Autodesk Inventor part; units mm, degrees
ref_plane "YZ Plane" through (0, 0, 0) normal (1, 0, 0) x (0, 1, 0)
ref_plane "XZ Plane" through (0, 0, 0) normal (0, 1, 0) x (-1, 0, 0)
ref_plane "XY Plane" through (0, 0, 0) normal (0, 0, 1) x (1, 0, 0)
sketch "Sketch1" plane through (0, 0, 0) normal (0, 0, 1) x (1, 0, 0)
  line L0 (10, -20) -> (-10, -20)
  line L1 (-10, -20) -> (-10, 20)
  line L2 (-10, 20) -> (10, 20)
  line L3 (10, 20) -> (10, -20)
  line L4 (10, -20) -> (-10, 20) construction
  line L5 (-10, -20) -> (10, 20) construction
  line L6 (0, -10) -> (0, 10) construction
  circle A0 centre (0, 10) radius 2.65
  circle A1 centre (0, -10) radius 2.65
  point P0 (0, 0)
  dimension "d0" = 40
  dimension "d1" = 20
  dimension "d2" = 20
  dimension "d3" = 5.3
extrude "Extrusion1" add sketch "Sketch1" along normal blind 3
ref_plane "Work Plane2" through (0, 0, -24) normal (0, 0, -1) x (-1, 0, 0)
sketch "Sketch2" plane through (0, 0, -24) normal (0, 0, -1) x (-1, 0, 0)
  circle A0 centre (18.05, -6.8) radius 1.65
  line L0 (18.05, -25.9) -> (18.05, -6.8) construction
  line L1 (4.6, -29) -> (20.7, -29)
  line L2 (4.6, 11.5) -> (4.6, -29)
  line L3 (20.7, 11.5) -> (4.6, 11.5)
  line L4 (20.7, -29) -> (20.7, 11.5)
  circle A1 centre (18.05, -25.9) radius 1.65
  line L5 (10, 20) -> (10, -20)
  line L6 (-10, 20) -> (10, 20)
  point P0 (0, 0)
  dimension "d8" = 40.5
  dimension "d9" = 16.1
  dimension "d10" = 19.1
  dimension "d11" = 3.3
  dimension "d12" = 3.3
  dimension "d13" = 2.65
  dimension "d14" = 3.1
  dimension "d15" = 8.05
  dimension "d19" = 26.8
extrude "Extrusion2" add sketch "Sketch2" against normal blind 3
sketch "Sketch4" plane through (0, 0, -21) normal (0, 0, 1) x (1, 0, 0)
  line L0 (-20.7, -14.85) -> (-4.6, -14.85)
  line L1 (-4.6, -14.85) -> (-4.6, -17.85)
  line L2 (-4.6, -17.85) -> (-20.7, -17.85)
  line L3 (-20.7, -17.85) -> (-20.7, -14.85)
  line L4 (-4.6, 1.5) -> (-20.7, 1.5)
  line L5 (-20.7, 1.5) -> (-20.7, -1.5)
  line L6 (-20.7, -1.5) -> (-4.6, -1.5)
  line L7 (-4.6, -1.5) -> (-4.6, 1.5)
  line L8 (-20.7, -16.35) -> (-4.6, -16.35) construction
  circle A0 centre (-18.05, -6.8) radius 1.65
  circle A1 centre (-18.05, -25.9) radius 1.65
  line L9 (-18.05, -6.8) -> (-18.05, -25.9) construction
  line L10 (-4.6, -29) -> (-4.6, 11.5)
  line L11 (-20.7, 11.5) -> (-20.7, -29)
  line L12 (-20.7, 0) -> (-4.6, 0) construction
  line L13 (-10, 20) -> (-10, -20)
  point P0 (0, 0)
  point P1 (-18.05, -16.35)
  point P2 (-10, 0)
  dimension "d20" = 3
sketch "Sketch5" plane through (0, 0, 0) normal (0, 0, -1) x (-1, 0, 0)
  line L0 (4.6, 1.5) -> (20.7, 1.5)
  line L1 (20.7, -1.5) -> (4.6, -1.5)
  line L2 (4.6, -17.85) -> (20.7, -17.85)
  line L3 (20.7, -14.85) -> (4.6, -14.85)
  line L4 (-10, 1.5) -> (10, 1.5)
  line L5 (10, 1.5) -> (10, -1.5)
  line L6 (10, -1.5) -> (-10, -1.5)
  line L7 (-10, -1.5) -> (-10, 1.5)
  line L8 (-10, -14.85) -> (10, -14.85)
  line L9 (10, -14.85) -> (10, -17.85)
  line L10 (10, -17.85) -> (-10, -17.85)
  line L11 (-10, -17.85) -> (-10, -14.85)
  line L12 (-10, -20) -> (-10, 20)
  line L13 (10, 20) -> (10, -20)
  point P0 (0, 0)
loft "Loft1" add profiles "Sketch4", "Sketch5" contours L5 L4 L13 L6 | L13 L4 L7 L6 / L0 L5 L1 L6 L7 L4
loft "Loft2" add profiles "Sketch4", "Sketch5" contours L0 L13 L2 L3 | L0 L1 L2 L13 / L9 L2 L10 L11 L8 L3
sketch "Sketch6" plane through (0, 0, -21) normal (0, 0, 1) x (1, 0, 0)
  line L0 (-20.7, 1.5) -> (-4.6, 1.5)
  line L1 (-4.6, 1.5) -> (-4.6, 11.5)
  line L2 (-4.6, 11.5) -> (-20.7, 11.5)
  line L3 (-20.7, 11.5) -> (-20.7, 1.5)
  point P0 (0, 0)
extrude "Extrusion3" cut sketch "Sketch6" against normal through all
properties part number "Soporte X"
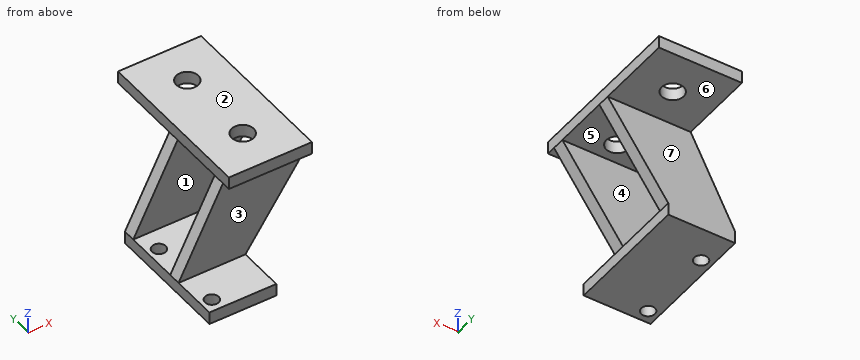
Could you check a few things on this model? Use its own coordinates, in mm. Face numbers are marked on the shaded views. A direction names the side the tool comes from. Coordinates: 2 decimals unless noted, no trailing zeros. Loops run counter-clockwise (first coordinate to the right, second up) from the corner with the lowest first, then second, coordinate; pieces in that order, holes last. Notation, with made-up numbers: (66, 78.5) -> (124, 78.5) arc R14 cw to (124, 101.5) -> close; hole circle Ø4 at (87.25, 77). An arc over 180 degrees is marked (long way). Answer in a Markdown table with one row per item.
(1) Imagine slicing it at C-C (y = -25.9). List the corners of the cut face in (x, z) for me, plus the area to 3 significant figures.
Results found:
| item | result |
|---|---|
| outline | (-20.7, -24) -> (-19.7, -24) -> (-19.7, -21) -> (-20.7, -21) -> close; (-16.4, -24) -> (-4.6, -24) -> (-4.6, -21) -> (-16.4, -21) -> close |
| area | 38.4 mm^2 |
(2) Will these pins go through, and if not, where does the flat tip stop? pin 1 Ø1.5 at (x, z) = (-7, -6) entering from +Y; pin 2 Ø1.5 at (x, z) = (1.5, 1.5) entering from -Y; pin 3 Ø4 at (x, y) = (-18.05, -25.9) entering from +Z; pin 4 Ø12 at (x, y) = (-17.5, -7.5) entering from -Z.
Results found:
| item | result |
|---|---|
| pin 1 | stops at y = 1.5 |
| pin 2 | stops at y = -20 |
| pin 3 | stops at z = -21 |
| pin 4 | stops at z = -24 |
(3) Imagine slicing it at D-D (z = -8.5). List the corners of the cut face in (x, y) for me, plus the area to 3 significant figures.
Results found:
| item | result |
|---|---|
| outline | (-14.33, -17.85) -> (4.09, -17.85) -> (4.09, -14.85) -> (-14.33, -14.85) -> close; (-14.33, -1.5) -> (4.09, -1.5) -> (4.09, 1.5) -> (-14.33, 1.5) -> close |
| area | 111 mm^2 |
(4) Imagine slicing it at B-B (x = -7.5). List the corners of the cut face in (y, z) for me, plus the area to 4 significant figures.
Results found:
| item | result |
|---|---|
| outline | (-29, -24) -> (1.5, -24) -> (1.5, 0) -> (20, 0) -> (20, 3) -> (-20, 3) -> (-20, 0) -> (-17.85, 0) -> (-17.85, -21) -> (-29, -21) -> close; hole (-14.85, -21) -> (-1.5, -21) -> (-1.5, 0) -> (-14.85, 0) -> close |
| area | 337.5 mm^2 |
(5) For the marked faces 1, 2 and 3, which set-ups out of +Z, -Z, +X, -X, +Y, -Y let a thin tool reach every point of the face, with its end or its side?
Results found:
| item | result |
|---|---|
| face 1 | +X, -X |
| face 2 | +Z, +X, -X, +Y, -Y |
| face 3 | +X, -X, -Y |
(6) If I drill on probe 1 along Y at (x, z) = (0, 1.85); probe 2 along Y at (x, z) = (-18.05, -21.7); probe 3 along Y at (x, z) = (-7.5, -4), over which ranges is the centre line in solid material (lowest first)?
Results found:
| item | result |
|---|---|
| probe 1 | y = -20 to -12.65, -7.35 to 7.35, 12.65 to 20 |
| probe 2 | y = -29 to -27.55, -24.25 to -8.45, -5.15 to 1.5 |
| probe 3 | y = -17.85 to -14.85, -1.5 to 1.5 |
(7) Thinking about a two-plate mould opening in Z: for the marked faces 4, 5, 6 and 7, which applies, released by +Z, released by -Z, zero draft, split by the parting line, or undercut?
Results found:
| item | result |
|---|---|
| face 4 | undercut |
| face 5 | undercut |
| face 6 | released by -Z |
| face 7 | zero draft |
(8) Imagine slicing it at A-A (y = -6.8). List the corners of the cut face in (x, z) for me, plus the area to 3 significant figures.
Results found:
| item | result |
|---|---|
| outline | (-20.7, -24) -> (-19.7, -24) -> (-19.7, -21) -> (-20.7, -21) -> close; (-16.4, -24) -> (-4.6, -24) -> (-4.6, -21) -> (-16.4, -21) -> close; (-10, 0) -> (10, 0) -> (10, 3) -> (-10, 3) -> close |
| area | 98.4 mm^2 |
